Autodesk Inventor part; units mm, degrees
ref_plane "YZ Plane" through (0, 0, 0) normal (1, 0, 0) x (0, 1, 0)
ref_plane "XZ Plane" through (0, 0, 0) normal (0, 1, 0) x (-1, 0, 0)
ref_plane "XY Plane" through (0, 0, 0) normal (0, 0, 1) x (1, 0, 0)
sketch "Sketch1" plane through (0, 0, 0) normal (1, 0, 0) x (0, 1, 0)
  line L0 (11, -5) -> (11, -5.0385)
  line L1 (10.8812, -5.1853) -> (0.604, -7.3697)
  line L2 (0, -6.8807) -> (0, -6.2052)
  line L3 (0.1464, -5.8517) -> (0.8517, -5.1464)
  line L4 (1.2052, -5) -> (11, -5)
  line L5 (0, 0) -> (10.4698, 0) construction
  arc A0 (0, -6.8807) -> (0.604, -7.3697) centre (0.5, -6.8807) ccw
  arc A1 (0.1464, -5.8517) -> (0, -6.2052) centre (0.5, -6.2052) ccw
  arc A2 (10.8812, -5.1853) -> (11, -5.0385) centre (10.85, -5.0385) ccw
  arc A3 (1.2052, -5) -> (0.8517, -5.1464) centre (1.2052, -5.5) ccw
  point P0 (11, -5.16)
  point P1 (0, -7.4981)
  point P2 (0, -5.9981)
  dimension "d0" = 11
  dimension "d1" = 12
  dimension "d2" = 5.16
  dimension "d3" = 5
  dimension "d4" = 1.5
  dimension "d6" = 45
  dimension "d7" = 7.4981
  dimension "d8" = 0.5
  dimension "d9" = 0.15
revolve "Revolution1" add sketch "Sketch1" angle 360 about axis through (0, 0, 0) along (0, 1, 0)
sketch "Sketch2" plane through (0, 0, 0) normal (0, 1, 0) x (-1, 0, 0)
  line L0 (0.5, -6.39) -> (-0.5, -6.39)
  line L1 (-0.5, -6.39) -> (-0.5, 0)
  line L2 (-0.5, 0) -> (0.5, 0)
  line L3 (0.5, 0) -> (0.5, -6.39)
  point P0 (0, 0)
  point P1 (0, 0)
  dimension "d11" = 1
  dimension "d12" = 6.39
extrude "Extrusion1" cut sketch "Sketch2" along normal through all
properties part number "Component 43(Engine Cone)"
Model file for the job. Use its own axes, mm. A direction names the side the tool comes from. Coordinates: 2 decimals unless noted, no trailing zeros. Order: outer loops, then holes, each group sorted by start corner. A loop starts at its lowest first (then second) coordinate and runs counter-clockwise, first axis right, second up. Notation, with made-up numbers: M 30,-6 L 50,-6 A7 cw 50,-2 Z; hole C 1.25,15.5 d11. An arc over 180 degrees is marked long. Return JSON: item names as keys, results as strings.
1. Tool access for faces 1 (the face through (-0.5, 4, -6)), 2 (the face through (0.225, 0.729, 5.264)): list every direction of +Z, -Z, +X, -X, +Y, -Y with a clear straight run to the whole face (end or side of a thin tool).
Ans:
{"face 1": "+Y, -Y", "face 2": "-Y"}
2. Saw through at D-D (y = 7.75). Give the cut face in (x, z), and give its area (3 significant figures).
Ans:
{"outline": "M -0.5,-5.83 L -0.5,-4.97 A5 cw long 0.5,-4.97 L 0.5,-5.83 A5.85 ccw long Z", "area": "28.2 mm^2"}
3. Flat gauge pins, fed straight in: pin 1 (4 mm diameter, centred on y = 3.5, z = -5.5, fed in from -X); pin 2 (1.5 mm diameter, centred on x = 3, y = 7.5, fed in from +Z); pin 3 (2 mm diameter, centred on y = 4, z = 1.5, fed in from -X); pin 4 (6 mm diameter, centred on x = 4, z = -2.5, fed in from -Y). Where does each tip first touch, or does it go through?
Ans:
{"pin 1": "x = -5.87", "pin 2": "z = 5.5", "pin 3": "x = -6.76", "pin 4": "y = 0"}
4. Pull direction X, two halves, no side cores. Call faces 3 (the face through (-5.906, 6.813, 1.312)), 4 (the face through (0, 3, -6.39)), 5 (the face through (-5, 0, 4)): +X half, -X half, draft (parallel to the pull), parting line (faces both ways), or undercut.
Ans:
{"face 3": "parting line", "face 4": "undercut", "face 5": "draft"}
5. Saw through at C-C (y = 4.5). Give the cut face in (x, z).
Ans:
{"outline": "C 0,0 d13.08; hole M -0.5,-6.39 L 0.5,-6.39 L 0.5,-4.97 A5 ccw long -0.5,-4.97 Z"}
6. Drill centre lines: probe 1 along X at (y, z) = (4.5, 0); probe 2 along X at (y, z) = (8, -4); probe 3 along Z at (x, y) = (4.25, 3.25). Where is each one in solid material? Low to high.
Ans:
{"probe 1": "-6.54 to -5, 5 to 6.54", "probe 2": "-4.2 to -3, 3 to 4.2", "probe 3": "-5.32 to -2.63, 2.63 to 5.32"}
